```python
from build123d import *

# Parameters (mm, degrees)
F0_W     = 20
F0_H     = 20
F1_DEPTH = 10
F2_W     = 12
F2_H     = 10
F3_DEPTH = 20
F5_DEPTH = 25
F6_D     = 5


with BuildPart() as f1:
    # F0 (on Right) → F1 (new body)
    with BuildSketch(Plane.YZ):
        with Locations((-4.31253016, -12.6576695228)):
            Rectangle(F0_W, F0_H)
    extrude(amount=F1_DEPTH)

    # F2 (on face) → F3 (join, through all)
    with BuildSketch(Plane.XZ.offset(14.31253016)):
        with Locations((-6, -12.6576695228)):
            Rectangle(F2_W, F2_H)
    extrude(amount=-F3_DEPTH)

    # F4 (on face) → F5 (cut)
    with BuildSketch(Plane.XY.offset(-7.6576695228)):
        with BuildLine():
            ThreePointArc((-12, -4.31253016), (-11.1449575543, -1.2255556274), (-8.8235294118, 0.9815874871))
            Line((-8.8235294118, 0.9815874871), (0, 5.68746984))
            Line((0, 5.68746984), (-12, 5.68746984))
            Line((-12, 5.68746984), (-12, -4.31253016))
        make_face()
        with BuildLine():
            ThreePointArc((-8.8235294118, -9.606647807), (-11.1449575543, -7.3995046925), (-12, -4.31253016))
            Line((-12, -4.31253016), (-12, -14.31253016))
            Line((-12, -14.31253016), (0, -14.31253016))
            Line((0, -14.31253016), (-8.8235294118, -9.606647807))
        make_face()
    extrude(amount=-F5_DEPTH, mode=Mode.SUBTRACT)

    # F6 (through all)
    with Locations(Plane.XY.offset(-7.6576695228)):
        with Locations((-6, -4.31253016)):
            Hole(F6_D / 2)


solid = f1.part
```
Verification items for the finished model (mm, model axes). A direction names the side the tool comes from. Coordinates: 2 decimals unless noted, no trailing zeros. Loops run counter-clockwise (first coordinate to the right, second up) from the corner with the lowest first, then second, coordinate; pieces in that order, holes last. Notation, with made-up numbers: (-31.5, 85.5) -> (-21.5, 85.5) arc R19 cw to (-21.5, 99.5) -> close; hole circle Ø9 at (42, 39). An arc over 180 degrees is marked (long way). Put each result on its own line as item: value.
1. Section check D-D, the plane x = -9.25. Record the boundary of the cut face in (y, z), then the cut area to 3 significant figures.
Result set:
outline: (-9.36, -17.66) -> (0.73, -17.66) -> (0.73, -7.66) -> (-9.36, -7.66) -> close
area: 101 mm^2
2. Section check A-A, the plane x = -4. Record the boundary of the cut face in (y, z).
Result set:
outline: (-12.18, -17.66) -> (-5.81, -17.66) -> (-5.81, -7.66) -> (-12.18, -7.66) -> close; (-2.81, -17.66) -> (3.55, -17.66) -> (3.55, -7.66) -> (-2.81, -7.66) -> close
3. Section check C-C, the plane y = -12. Record the boundary of the cut face in (x, z).
Result set:
outline: (-4.34, -17.66) -> (0, -17.66) -> (0, -22.66) -> (10, -22.66) -> (10, -2.66) -> (0, -2.66) -> (0, -7.66) -> (-4.34, -7.66) -> close
4. Section check B-B, the plane z = -11.5. Record the boundary of the cut face in (x, y).
Result set:
outline: (-8.82, -9.61) -> (0, -14.31) -> (10, -14.31) -> (10, 5.69) -> (0, 5.69) -> (-8.82, 0.98) arc R6 ccw to start; hole circle Ø5 at (-6, -4.31)
5. Thickness scan on line 1 (Z direction, x = -7.5, y = -6.75); line 2 (X direction, y = -6.5, z = -4); line 3 (Y direction, x = -7.25, z = -9.5). Record the ranges inside material, lowest first.
Result set:
line 1: z = -17.66 to -7.66
line 2: x = 0 to 10
line 3: y = -10.45 to -6.48, -2.15 to 1.82
6. Gauge pin test, flat ends, axial feed: P1, Ø2.5, axis at y = -1.5, z = -21, coming from the -X side; P2, Ø2, axis at x = -6, y = -3, coming from the -Z side; P3, Ø5, axis at x = -8, y = 1.5, coming from the +Z side; P4, Ø3, axis at y = -7.5, z = -7.5, coming from the -X side. Record the tip position at first contact, or that the pin passes through.
Result set:
P1: stops at x = 0
P2: passes through
P3: stops at z = -7.66
P4: stops at x = -11.76
7. Mould release check, pull along Z, two halves, no side actions. Record for faces 1 (the face through (-4.35, -11.993, -12.588)), 2 (the face through (5, -4, -22.658)), 3 (the face through (-3, -4, -7.658)): pulls with the +Z half, pulls with the -Z half, needs draft (parallel to the pull), parting line crosses it, or undercut.
Result set:
face 1: needs draft
face 2: pulls with the -Z half
face 3: pulls with the +Z half
8. Tool access check on faces 4 (the face through (-3, -4, -17.658)), 5 (the face through (5, -4, -2.658)), 6 (the face through (0, -4, -5)). Record the directions out of +Z, -Z, +X, -X, +Y, -Y that give a thin tool (end or side, any length) a straight path to the whole face; none if there is none.
Result set:
face 4: -Z, -X, +Y, -Y
face 5: +Z, +X, -X, +Y, -Y
face 6: +Z, -X, +Y, -Y
